CAD build for the part. Positions are in the model's coordinates, mm. A direction names the side the tool comes from. Coordinates: 2 decimals unless noted, no trailing zeros. Write each loop counter-clockwise with the first axis right and the second up, starting at its lowest first coordinate (ties: lowest second). Pieces come first, ordered by that corner, then holes. Notation, with made-up numbers: M 2,-30.5 L 23,-30.5 A9 ccw 23,-26.5 Z; hole C -36.5,-5.5 d9. An arc over 180 degrees is marked long. Answer as CSV lines item,"result". Start each with the question number.
```python
from build123d import *

# Parameters (mm, degrees)
SKETCH1_W           = 58.636614691
SKETCH1_H           = 33.890307345
SKETCH1_R           = 1.6129
SKETCH1_W_2         = 5.842
SKETCH1_H_2         = 10.414
BOSS_EXTRUDE1_DEPTH = 2.032
SKETCH2_W           = 31.75
SKETCH2_H           = 21.190307345
CUT_EXTRUDE1_DEPTH  = 68.756435402
FILLET1_R           = 5.08


with BuildPart() as part:
    # Sketch1 → Boss-Extrude1 (new body)
    with BuildSketch(Plane(origin=(0, 0, 0), x_dir=(1, 0, 0), z_dir=(0, 1, 0))):
        with Locations((29.318307346, 16.945153673)):
            Rectangle(SKETCH1_W, SKETCH1_H)
        with Locations(Location((19.793307345, 9.525, 0), (0, 0, 270))):
            Circle(SKETCH1_R, mode=Mode.SUBTRACT)
        with Locations(Location((19.793307345, 3.175, 0), (0, 0, 270))):
            Circle(SKETCH1_R, mode=Mode.SUBTRACT)
        with Locations(Location((38.843307345, 3.175, 0), (0, 0, 90))):
            Circle(SKETCH1_R, mode=Mode.SUBTRACT)
        with Locations(Location((38.843307345, 9.525, 0), (0, 0, 90))):
            Circle(SKETCH1_R, mode=Mode.SUBTRACT)
        with Locations((6.096, 25.508307345)):
            Rectangle(SKETCH1_W_2, SKETCH1_H_2, mode=Mode.SUBTRACT)
        with Locations((52.540614691, 25.508307345)):
            Rectangle(SKETCH1_W_2, SKETCH1_H_2, mode=Mode.SUBTRACT)
    extrude(amount=BOSS_EXTRUDE1_DEPTH)

    # Sketch2 → Cut-Extrude1 (cut, through all)
    with BuildSketch(Plane(origin=(0, 2.032, 0), x_dir=(1, 0, 0), z_dir=(0, 1, 0))):
        with Locations((29.318307345, 23.295153673)):
            Rectangle(SKETCH2_W, SKETCH2_H)
        Polygon((0, 16.945153673), (15.24, 0), (0, 0), align=None)
        Polygon((43.396614691, 0), (58.636614691, 0), (58.636614691, 16.945153673), align=None)
    extrude(amount=-CUT_EXTRUDE1_DEPTH, mode=Mode.SUBTRACT)

    # Fillet1
    fillet1_edges = [part.edges().sort_by_distance(p)[0] for p in [
        (43.396614691, 1.016, 0),
        (58.636614691, 1.016, -16.945153673),
        (0, 1.016, -16.945153673),
        (15.24, 1.016, 0),
        (0, 1.016, -33.890307345),
        (58.636614691, 1.016, -33.890307345),
        (13.443307345, 1.016, -33.890307345),
        (45.193307345, 1.016, -33.890307345),
        (45.193307345, 1.016, -12.7),
        (13.443307345, 1.016, -12.7),
    ]]
    fillet(fillet1_edges, radius=FILLET1_R)


solid = part.part
```
1) Tool access for faces 4 (the cylindrical face through (57.11, 1.03, -32.44)), 5 (the cylindrical face through (43.666, 1.002, -14.149)), 6 (the flat face through (3.175, 1, -25)): list every direction of +Z, -Z, +X, -X, +Y, -Y with a clear straight run to the whole face (end or side of a thin tool).
2) Band-saw the part on B-B, the plane x = 51.5. List the corners of the cut face in (y, z).
3) Probe L1, parallel to X at y = 0.85, z = -29 (3 decimals); L2, parallel to Z at x = 19, y = 0.65; L3, parallel to X at y = 1.5, z = -20. List the from-to ranges inside material, lowest first. Write a range as [from, to].
4) Band-saw the part on A-A, the plane z = -21. List the corners of the cut face in (x, y) (3 decimals), plus the area to 3 significant figures.
5) Band-saw the part on D-D, the plane z = -9. List the corners of the cut face in (x, y).
6) Pin check, flat tips, straight feed: P1, Ø1, axis at x = 5.5, y = 1, coming from the +Z side; P2, Ø2.5, axis at x = 38.84, z = -3.18, coming from the -Y side; P3, Ø6, axis at x = 22, z = -6.5, coming from the -Y side; P4, Ø1, axis at x = 34.5, y = 1, coming from the -Z side. Stop position of each tip, or through.
7) Two-plate mould, pull along Z, no slides. Class faces 1 (the cylindrical face through (37.48, 1, -10.39)), 2 (the flat face through (29, 1, -12.7)), 3 (the cylindrical face through (58.31, 1, -17.1)): pulls with the +Z half, pulls with the -Z half, needs draft (parallel to the pull), parting line crosses it, or undercut.
8) Band-saw the part on C-C, the plane y = 1.55. State how many separate pieces and enclosed holes the cut face has, plus the area to 3 significant figures.
Result sheet:
1,face 4,"-Z, +X, +Y, -Y"
1,face 5,"-Z, +Y, -Y"
1,face 6,"+Y, -Y"
2,outline,"M 0,-33.89 L 2.03,-33.89 L 2.03,-30.72 L 0,-30.72 Z; M 0,-20.3 L 2.03,-20.3 L 2.03,-9.01 L 0,-9.01 Z"
3,L1,"x = [0.004, 3.175], [9.017, 13.44], [45.197, 49.62], [55.462, 58.633]"
3,L2,"z = [-12.7, -10.93], [-8.12, -4.58], [-1.77, 0]"
3,L3,"x = [0, 13.44], [45.19, 58.64]"
4,outline,"M 0,0 L 3.175,0 L 3.175,2.032 L 0,2.032 Z; M 9.017,0 L 13.443,0 L 13.443,2.032 L 9.017,2.032 Z; M 45.193,0 L 49.62,0 L 49.62,2.032 L 45.193,2.032 Z; M 55.462,0 L 58.637,0 L 58.637,2.032 L 55.462,2.032 Z"
4,area,"30.9 mm²"
5,outline,"M 7.15,0 L 18.27,0 L 18.27,2.03 L 7.15,2.03 Z; M 21.32,0 L 37.32,0 L 37.32,2.03 L 21.32,2.03 Z; M 40.37,0 L 51.49,0 L 51.49,2.03 L 40.37,2.03 Z"
6,P1,"stops at z = -10.27"
6,P2,"passes through"
6,P3,"stops at y = 0"
6,P4,"stops at z = -12.7"
7,face 1,"undercut"
7,face 2,"pulls with the -Z half"
7,face 3,"pulls with the +Z half"
8,separate pieces,"1"
8,enclosed holes,"6"
8,area,"888 mm²"
